The figure shows three views and two pictorial views of one solid part (mm, origin at its lowest corner). Answer the questions. Round coordinates to 2 decimals unless told otherwise and drop trailing zeros. Write each loop counter-clockwise with the first axis right and the second up, starting at its lowest first coordinate (ties: lowest second). Pieces come first, ordered by that corner, then holes. Notation, with made-up numbers: M 81,79.5 L 110,79.5 A19 cw 110,111.5 Z; hole C 63.5,-39 d1. An arc over 180 degrees is marked long. Answer in a Markdown table with one row per item.
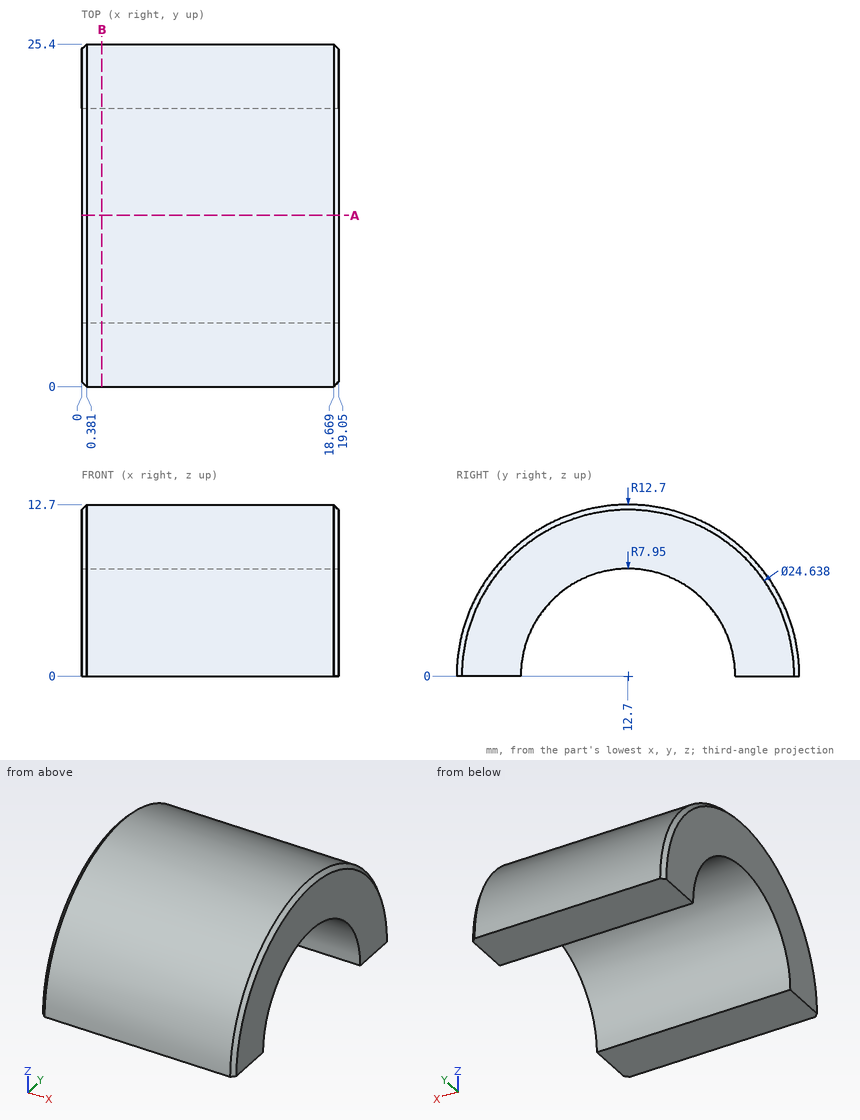
1. Consider line 1 along Y through (x, z) = (9.75, 3); line 2 along Y through (x, z) = (4.5, 5.5); line 3 along Z through (x, y) = (17, 12.5). Determine where each line is inside the solid, lowest interval first. Write a range as from..to.
Calculated:
| item | result |
|---|---|
| line 1 | y = 0.36..5.34, 20.06..25.04 |
| line 2 | y = 1.25..6.96, 18.44..24.15 |
| line 3 | z = 7.95..12.7 |
2. The part is cut by section B-B (x = 1.5). Determine the outline of the cut face in (y, z).
Calculated:
| item | result |
|---|---|
| outline | M 0,0 L 4.75,0 A7.95 cw 20.65,0 L 25.4,0 A12.7 ccw Z |
3. Given pin 1 (8 mm diameter, centred on x = 13.5, y = 6, fed in from +Z); pin 2 (3 mm diameter, centred on x = 6, y = 18.5, fed in from +Z); pin 3 (6 mm diameter, centred on x = 8.5, z = 7.5, fed in from +Y), each flat-ended and moving along its own axis, determine where each tip first touches the part or whether it passes through.
Calculated:
| item | result |
|---|---|
| pin 1 | stops at z = 12.41 |
| pin 2 | stops at z = 11.95 |
| pin 3 | stops at y = 24.58 |
4. The part is cut by section A-A (y = 12.7). Determine the outline of the cut face in (x, z).
Calculated:
| item | result |
|---|---|
| outline | M 0,7.95 L 19.05,7.95 L 19.05,12.32 L 18.67,12.7 L 0.38,12.7 L 0,12.32 Z |
